Can you work these out from the model? Positions are in its coordinate system, mm. Round coordinates to 2 decimals unless told otherwise and drop trailing zeros. Loops run counter-clockwise (first coordinate to the right, second up) from the corner with the lowest first, then second, coordinate; pieces in that order, holes last.
(1) Will these pins go through, and if not, where does the flat tip stop? pin 1 Ø7.5 at (x, z) = (300, 0) entering from +Y; pin 2 Ø0.6 at (x, y) = (152, 8.5) entering from -Z.
(2) If I drill on line 1 along Y through (x, z) = (209, -8.25); line 2 along Z through (x, y) = (300, 8); line 3 along Z through (x, y) = (180, 1.3), over which ranges is the centre line in solid material (lowest first)?
(3) I want a section at A-A on x = 104. Write out the boundary of the cut face in (y, z), plus the area to 3 significant figures.
from build123d import *

# Parameters (mm, degrees)
SKETCH1_W                                    = 20
SKETCH1_H                                    = 11
BOSS_EXTRUDE1_DEPTH                          = 400
CUT_EXTRUDE2_DEPTH                           = 401.276154673
CBORE_FOR_SOCKET_HEAD_CAP_SCREW1_D           = 6
CBORE_FOR_SOCKET_HEAD_CAP_SCREW1_CBORE_D     = 9.5
CBORE_FOR_SOCKET_HEAD_CAP_SCREW1_CBORE_DEPTH = 5.5
LPATTERN1_COUNT                              = 7
LPATTERN1_PITCH                              = 60
CHAMFER1_SIZE                                = 0.3
CHAMFER2_SIZE                                = 0.5


with BuildPart() as part:
    # Sketch1 → Boss-Extrude1 (new body)
    with BuildSketch(Plane(origin=(-30.5, 0, 0), x_dir=(0, 0, -1), z_dir=(1, 0, 0))):
        with Locations((0, 5.5)):
            Rectangle(SKETCH1_W, SKETCH1_H)
    extrude(amount=BOSS_EXTRUDE1_DEPTH)

    # Sketch3 → Cut-Extrude2 (cut, through all)
    with BuildSketch(Plane(origin=(-30.5, 0, 0), x_dir=(0, 0, -1), z_dir=(1, 0, 0))):
        with BuildLine():
            Line((10, 10.451039482), (9.455259378, 10.141421591))
            ThreePointArc((9.455259378, 10.141421591), (8.943868436, 9.701092928), (8.637115571, 9.1))
            Line((8.637115571, 9.1), (7.5, 9.1))
            Line((7.5, 9.1), (7.5, 7.9))
            Line((7.5, 7.9), (8.64, 7.9))
            ThreePointArc((8.64, 7.9), (8.939788863, 7.314120259), (9.434780564, 6.880401858))
            Line((9.434780564, 6.880401858), (10, 6.548960518))
            Line((10, 6.548960518), (10, 10.451039482))
        make_face()
        with BuildLine():
            Line((-10, 10.451039482), (-10, 6.548960518))
            Line((-10, 6.548960518), (-9.434780564, 6.880401858))
            ThreePointArc((-9.434780564, 6.880401858), (-8.939788863, 7.314120259), (-8.64, 7.9))
            Line((-8.64, 7.9), (-7.5, 7.9))
            Line((-7.5, 7.9), (-7.5, 9.1))
            Line((-7.5, 9.1), (-8.637115571, 9.1))
            ThreePointArc((-8.637115571, 9.1), (-8.943868436, 9.701092928), (-9.455259378, 10.141421591))
            Line((-9.455259378, 10.141421591), (-10, 10.451039482))
        make_face()
    extrude(amount=CUT_EXTRUDE2_DEPTH, mode=Mode.SUBTRACT)

    # CBORE for Socket Head Cap Screw1 (through all)
    with Locations(Plane(origin=(0, 11, 0), x_dir=(1, 0, 0), z_dir=(0, 1, 0))):
        with Locations((0, 0)):
            cbore_for_socket_head_cap_screw1 = CounterBoreHole(CBORE_FOR_SOCKET_HEAD_CAP_SCREW1_D / 2, CBORE_FOR_SOCKET_HEAD_CAP_SCREW1_CBORE_D / 2, CBORE_FOR_SOCKET_HEAD_CAP_SCREW1_CBORE_DEPTH)

    # LPattern1: CBORE for Socket Head Cap Screw1 ×7
    with Locations(*[(i * LPATTERN1_PITCH, 0, 0) for i in range(1, LPATTERN1_COUNT)]):
        add(cbore_for_socket_head_cap_screw1, mode=Mode.SUBTRACT)

    # Chamfer1
    chamfer1_edges = [part.edges().sort_by_distance(p)[0] for p in [
        (169.5, 11, 10),
        (169.5, 11, -10),
    ]]
    chamfer(chamfer1_edges, length=CHAMFER1_SIZE)

    # Chamfer2
    chamfer2_edges = [part.edges().sort_by_distance(p)[0] for p in [
        (169.5, 0, -10),
        (169.5, 0, 10),
    ]]
    chamfer(chamfer2_edges, length=CHAMFER2_SIZE)


solid = part.part
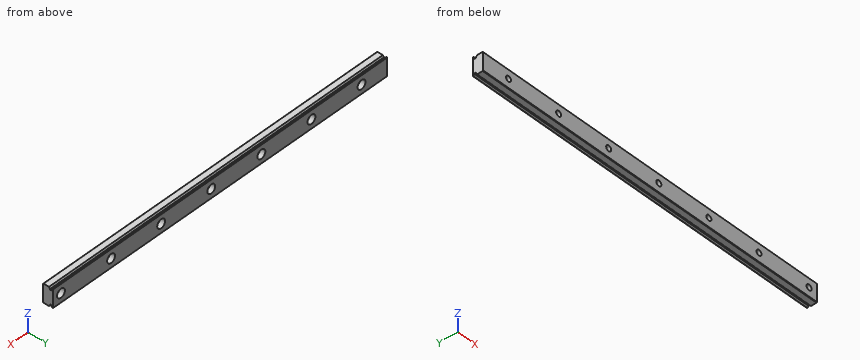
Filled sheet:
1. pin 1: stops at y = 5.5
1. pin 2: stops at z = -7.5
2. line 1: y = 0 to 7.9, 9.1 to 11
2. line 2: z = -7.5 to -4.75, 4.75 to 7.5
2. line 3: z = -10 to -3, 3 to 10
3. outline: (0, -9.5) - (0.5, -10) - (6.55, -10) - (6.88, -9.43) arc R1.75 cw to (7.9, -8.64) - (7.9, -7.5) - (9.1, -7.5) - (9.1, -8.64) arc R1.75 cw to (10.14, -9.46) - (10.45, -10) - (10.7, -10) - (11, -9.7) - (11, 9.7) - (10.7, 10) - (10.45, 10) - (10.14, 9.46) arc R1.75 cw to (9.1, 8.64) - (9.1, 7.5) - (7.9, 7.5) - (7.9, 8.64) arc R1.75 cw to (6.88, 9.43) - (6.55, 10) - (0.5, 10) - (0, 9.5) - close
3. area: 209 mm2
